```python
from build123d import *

# Parameters (mm, degrees)
SKETCH1_W          = 101.6
SKETCH1_H          = 76.2
BASE_DEPTH         = 6.35
TUBE_NOTCH_DEPTH   = 64.816710194
MOUNTING_HOLES_D   = 4.4958
SKETCH8_W          = 76.2
SKETCH8_H          = 38.1
WHEEL_CUTOUT_DEPTH = 64.816710194
FILLET1_R          = 6.35
FILLET2_R          = 9.525
CUT_EXTRUDE1_DEPTH = 64.816710194
FILLET3_R          = 3.175


with BuildPart() as part:
    # Sketch1 → Base (new body)
    with BuildSketch(Plane(origin=(0, 0, 0), x_dir=(1, 0, 0), z_dir=(0, 1, 0))):
        Rectangle(SKETCH1_W, SKETCH1_H)
    extrude(amount=BASE_DEPTH)

    # Sketch2 → Tube notch (cut, through all)
    with BuildSketch(Plane(origin=(0, 6.35, 0), x_dir=(1, 0, 0), z_dir=(0, 1, 0))):
        Polygon((-44.45, 38.1), (0, 14.855181866), (44.45, 38.1), align=None)
    extrude(amount=-TUBE_NOTCH_DEPTH, mode=Mode.SUBTRACT)

    # Mounting holes (through all)
    with Locations(Plane(origin=(0, 6.35, 0), x_dir=(1, 0, 0), z_dir=(0, 1, 0))):
        with Locations((-44.45, -6.35), (-44.45, -31.75), (44.45, -31.75), (44.45, -6.35)):
            Hole(MOUNTING_HOLES_D / 2)

    # Sketch8 → Wheel cutout (cut, through all)
    with BuildSketch(Plane(origin=(0, 6.35, 0), x_dir=(1, 0, 0), z_dir=(0, 1, 0))):
        with Locations((0, -19.05)):
            Rectangle(SKETCH8_W, SKETCH8_H)
    extrude(amount=-WHEEL_CUTOUT_DEPTH, mode=Mode.SUBTRACT)

    # Fillet1
    # the kernel refuses this fillet: 6.35 mm, written as the material it adds along each edge
    with BuildSketch(Plane(origin=(38.1, 6.35, 0), x_dir=(0, 0, 1), z_dir=(0, -1, 0))) as fillet1_piece_1:
        with BuildLine():
            CenterArc((FILLET1_R, FILLET1_R), FILLET1_R, 180, 90)
            Line((0, FILLET1_R), (0, 0))
            Line((0, 0), (FILLET1_R, 0))
        make_face()
    extrude(amount=6.35)
    with BuildSketch(Plane(origin=(-38.1, 6.35, 0), x_dir=(0, 0, 1), z_dir=(0, -1, 0))) as fillet1_piece_2:
        with BuildLine():
            CenterArc((FILLET1_R, -FILLET1_R), FILLET1_R, 90, 90)
            Line((0, -FILLET1_R), (0, 0))
            Line((0, 0), (FILLET1_R, 0))
        make_face()
    extrude(amount=6.35)
    # the kernel refuses this fillet: 6.35 mm, written as the material it takes off along each edge
    with BuildSketch(Plane(origin=(-50.8, -15.875, 38.1), x_dir=(1, 0, 0), z_dir=(0, 1, 0)), Plane(origin=(50.8, -15.875, -38.1), x_dir=(-1, 0, 0), z_dir=(0, 1, 0)), Plane(origin=(50.8, -15.875, 38.1), x_dir=(0, 0, -1), z_dir=(0, 1, 0)), Plane(origin=(-38.1, 22.225, 38.1), x_dir=(-1, 0, 0), z_dir=(0, -1, 0)), Plane(origin=(-50.8, -15.875, -38.1), x_dir=(0, 0, 1), z_dir=(0, 1, 0))) as fillet1_2_piece_1:
        with BuildLine():
            CenterArc((FILLET1_R, FILLET1_R), FILLET1_R, 180, 90)
            Line((0, FILLET1_R), (0, 0))
            Line((0, 0), (FILLET1_R, 0))
        make_face()
    extrude(amount=38.1, mode=Mode.SUBTRACT)
    with BuildSketch(Plane(origin=(-44.45, 10.250302923, -38.1), x_dir=(-1, 0, 0), z_dir=(0, -1, 0)), Plane(origin=(44.45, 10.250302923, -38.1), x_dir=(-0.8861469338573508, 0, 0.46340437159700587), z_dir=(0, -1, 0))) as fillet1_2_piece_2:
        with BuildLine():
            CenterArc((FILLET1_R * 0.245688373095, -FILLET1_R), FILLET1_R, 90, 27.607004509)
            Line((-FILLET1_R * 0.217715998502, -FILLET1_R * 0.113853066143), (0, 0))
            Line((0, 0), (FILLET1_R * 0.245688373095, 0))
        make_face()
    extrude(amount=14.150605846, mode=Mode.SUBTRACT)
    with BuildSketch(Plane(origin=(38.1, 22.225, 38.1), x_dir=(1, 0, 0), z_dir=(0, -1, 0))) as fillet1_2_piece_3:
        with BuildLine():
            CenterArc((FILLET1_R, -FILLET1_R), FILLET1_R, 90, 90)
            Line((0, -FILLET1_R), (0, 0))
            Line((0, 0), (FILLET1_R, 0))
        make_face()
    extrude(amount=38.1, mode=Mode.SUBTRACT)

    # Fillet2
    fillet2_edges = [part.edges().sort_by_distance(p)[0] for p in [
        (0, 3.175, -14.855181866),
    ]]
    fillet(fillet2_edges, radius=FILLET2_R)

    # Sketch9 → Cut-Extrude1 (cut, through all)
    with BuildSketch(Plane(origin=(0, 6.35, 0), x_dir=(1, 0, 0), z_dir=(0, 1, 0))):
        Polygon((-44.45, 6.35), (-44.45, 30.934145493), (-3.175, 9.349671511), (-3.175, 6.35), align=None)
        Polygon((3.175, 9.349671511), (44.45, 30.934145493), (44.45, 6.35), (3.175, 6.35), align=None)
    extrude(amount=-CUT_EXTRUDE1_DEPTH, mode=Mode.SUBTRACT)

    # Fillet3
    # the kernel refuses this fillet: 3.175 mm, written as the material it adds along each edge
    with BuildSketch(Plane(origin=(-44.45, 6.35, -6.35), x_dir=(1, 0, 0), z_dir=(0, -1, 0))) as fillet3_piece_1:
        with BuildLine():
            CenterArc((FILLET3_R, -FILLET3_R), FILLET3_R, 90, 90)
            Line((0, -FILLET3_R), (0, 0))
            Line((0, 0), (FILLET3_R, 0))
        make_face()
    extrude(amount=6.35)
    with BuildSketch(Plane(origin=(-3.175, 6.35, -9.349671511), x_dir=(0, 0, 1), z_dir=(0, -1, 0))) as fillet3_piece_2:
        with BuildLine():
            CenterArc((FILLET3_R * 0.605537984618, FILLET3_R), FILLET3_R, 207.607004509, 62.392995491)
            Line((-FILLET3_R * 0.28060894924, FILLET3_R * 0.536595628403), (0, 0))
            Line((0, 0), (FILLET3_R * 0.605537984618, 0))
        make_face()
    extrude(amount=6.35)
    with BuildSketch(Plane(origin=(-3.175, 6.35, -6.35), x_dir=(-1, 0, 0), z_dir=(0, -1, 0)), Plane(origin=(44.45, 6.35, -6.35), x_dir=(-1, 0, 0), z_dir=(0, -1, 0)), Plane(origin=(3.175, 6.35, -6.35), x_dir=(0, 0, -1), z_dir=(0, -1, 0))) as fillet3_piece_3:
        with BuildLine():
            CenterArc((FILLET3_R, FILLET3_R), FILLET3_R, 180, 90)
            Line((0, FILLET3_R), (0, 0))
            Line((0, 0), (FILLET3_R, 0))
        make_face()
    extrude(amount=6.35)
    with BuildSketch(Plane(origin=(3.175, 6.35, -9.349671511), x_dir=(0, 0, 1), z_dir=(0, -1, 0))) as fillet3_piece_4:
        with BuildLine():
            CenterArc((FILLET3_R * 0.605537984618, -FILLET3_R), FILLET3_R, 90, 62.392995491)
            Line((-FILLET3_R * 0.28060894924, -FILLET3_R * 0.536595628403), (0, 0))
            Line((0, 0), (FILLET3_R * 0.605537984618, 0))
        make_face()
    extrude(amount=6.35)
    with BuildSketch(Plane(origin=(44.45, 6.35, -30.934145493), x_dir=(0, 0, 1), z_dir=(0, -1, 0)), Plane(origin=(-44.45, 6.35, -30.934145493), x_dir=(0.8861469338573508, 0, 0.463404371597006), z_dir=(0, -1, 0))) as fillet3_piece_5:
        with BuildLine():
            CenterArc((FILLET3_R * 1.65142406489, FILLET3_R), FILLET3_R, 152.392995491, 117.607004509)
            Line((FILLET3_R * 0.765277131029, FILLET3_R * 1.4634043716), (0, 0))
            Line((0, 0), (FILLET3_R * 1.65142406489, 0))
        make_face()
    extrude(amount=6.35)


solid = part.part
```
CAD build for the part. Positions are in the model's coordinates, mm. A direction names the side the tool comes from. Round coordinates to 2 decimals unless told otherwise and drop trailing zeros. Order: outer loops, then holes, each group sorted by start corner. A loop starts at its lowest first (then second) coordinate and runs counter-clockwise, first axis right, second up. Notation, with made-up numbers: (-29.5, 15) - (-18.5, 15) arc R29 ccw to (-18.5, 51) - close; hole circle Ø6 at (-32.75, -6.5). An arc over 180 degrees is marked (long way). Answer as CSV lines item,"result". Start each with the question number.
1. Saw through at B-B, the plane x = -28.5. Write the cut outline in (y, z), and give its area (3 significant figures).
2. Saw through at D-D, the plane z = -22.5. Write the cut outline in (x, y), and give its area (3 significant figures).
3. Pull direction Z, two halves, no side cores. Call faces 1 (the face through (-42.67, 3.13, 7.72)), 2 (the face through (0, 3, 0)), 3 (the face through (49.25, 3.13, -35.91)): +Z half, -Z half, draft (parallel to the pull), parting line (faces both ways), or undercut.
4. Drill centre lines: L1, parallel to X at y = 4.25, z = 31.75; L2, parallel to X at y = 4.75, z = -7.5; L3, parallel to X at y = 3, z = 7.5. Where is each one in solid material? Low to high. Write a range as [from, to].
5. Saw through at C-C, the plane y = 3.25. Count the separate pieces of the cut face and the enclosed holes in it, and give its area (3 significant figures).
6. Saw through at A-A, the plane z = 25.5. Write the cut outline in (x, y).
7. Pin check, flat tips, straight feed: pin 1 (1.9 mm diameter, centred on x = -15.5, y = 3, fed in from -Z); pin 2 (1.5 mm diameter, centred on x = 3.5, y = 3.5, fed in from -Z); pin 3 (2 mm diameter, centred on x = 29.5, y = 4, fed in from -Z). Stop position of each tip, or through.
8. Tool access for faces 4 (the face through (38.1, 3, 19)), 5 (the face through (43.54, 3.22, -7.3)), 6 (the face through (44.103, 3.219, -37.807)), 7 (the face through (4, 6.35, -5)): list every direction of +Z, -Z, +X, -X, +Y, -Y with a clear straight run to the whole face (end or side of a thin tool).
Model answer:
1,outline,"(0, -29.76) - (6.35, -29.76) - (6.35, -22.59) - (0, -22.59) - close; (0, -6.35) - (6.35, -6.35) - (6.35, 0) - (0, 0) - close"
1,area,"85.8 mm²"
2,outline,"(-50.8, 0) - (-44.45, 0) - (-44.45, 6.35) - (-50.8, 6.35) - close; (-28.32, 0) - (-14.62, 0) - (-14.62, 6.35) - (-28.32, 6.35) - close; (14.62, 0) - (28.32, 0) - (28.32, 6.35) - (14.62, 6.35) - close; (44.45, 0) - (50.8, 0) - (50.8, 6.35) - (44.45, 6.35) - close"
2,area,"255 mm²"
3,face 1,"undercut"
3,face 2,"+Z half"
3,face 3,"-Z half"
4,L1,"x = [-50.8, -46.7], [-42.2, -38.1], [38.1, 42.2], [46.7, 50.8]"
4,L2,"x = [-50.8, -43.72], [-3.9, 3.9], [43.72, 50.8]"
4,L3,"x = [-50.8, -46.38], [-42.52, -38.1], [38.1, 42.52], [46.38, 50.8]"
5,separate pieces,"1"
5,enclosed holes,"6"
5,area,"2,590 mm²"
6,outline,"(-50.8, 0) - (-38.1, 0) - (-38.1, 6.35) - (-50.8, 6.35) - close; (38.1, 0) - (50.8, 0) - (50.8, 6.35) - (38.1, 6.35) - close"
7,pin 1,"stops at z = -23.46"
7,pin 2,"stops at z = -17.08"
7,pin 3,"stops at z = -30.8"
8,face 4,"+Z, +Y, -Y"
8,face 5,"+Y, -Y"
8,face 6,"-Z, +Y, -Y"
8,face 7,"+Z, -Z, +X, -X, +Y"
